Can you work these out from the model? Positions are in its coordinate system, mm. Give positions to 0.01 mm unless a question says otherwise; leave off trailing zeros. Loops run counter-clockwise (first coordinate to the right, second up) from the corner with the lowest first, then second, coordinate; pieces in that order, holes last. Notation, with made-up numbers: M 58,27.5 L 74,27.5 A9 ccw 74,32.5 Z; hole C -1.75,83.25 d7. An arc over 180 degrees is marked long. One line per item, written item: value. Start each with the question number.
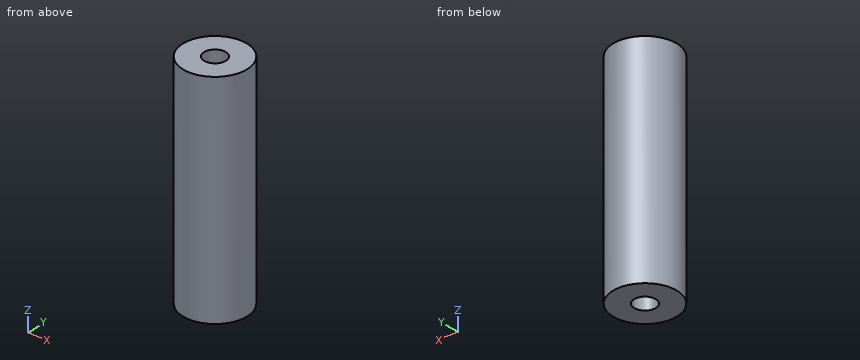
from build123d import *

# Parameters (mm, degrees)
SKETCH_2_W             = 43
SKETCH_2_H             = 12.5
HOLE_WIZARD_M101_D     = 8.5
HOLE_WIZARD_M101_DEPTH = 27.5
HOLE_WIZARD_M101_TIP   = 2.553657631


with BuildPart() as part:
    # Эскиз2 → Повернуть1 (revolve)
    with BuildSketch(Plane(origin=(0, 0, 0), x_dir=(0, 0, -1), z_dir=(1, 0, 0))):
        with Locations((21.5, 6.25)):
            Rectangle(SKETCH_2_W, SKETCH_2_H)
    revolve(axis=Axis((0, 0, 0), (0, 0, -1)))

    # Отверстие обработанное метчиком M101
    with Locations(Plane(origin=(0, 0, -43), x_dir=(-1, 0, 0), z_dir=(0, 0, -1))):
        with Locations((0, 0)):
            Hole(HOLE_WIZARD_M101_D / 2, depth=HOLE_WIZARD_M101_DEPTH)
            with Locations((0, 0, -(HOLE_WIZARD_M101_DEPTH + HOLE_WIZARD_M101_TIP / 2))):  # 118° drill point
                Cone(0, HOLE_WIZARD_M101_D / 2, HOLE_WIZARD_M101_TIP, mode=Mode.SUBTRACT)

    # Зеркальное отражение1: part across plane


with BuildPart() as part_1:
    add(part.part)
    add(part.part.mirror(Plane(origin=(0, 0, 0), x_dir=(1, 0, 0), z_dir=(0, 0, -1))))


solid = part_1.part
Q1. If we section it at B-B, the plane z = 24: Write out the boundary of the cut face in (x, y).
Q2. If we section it at D-D, the plane x = -9: Write out the boundary of the cut face in (y, z), plus the area to 3 significant figures.
Q3. I need wall thicknesses on line 1 along X through (y, z) = (0, 33); line 2 along X through (y, z) = (3.25, -32); line 3 along Y through (x, z) = (-0.5, 3.5). Which ranges of each line are inside material? Lowest first, please.
Q4. If we section it at A-A, the plane z = -1.5: Write out the boundary of the cut face in (x, y), plus the area to 3 significant figures.
Q5. For P1, Ø10, axis at x = 7, z = -8.5, coming from the -Y side; P2, Ø10, axis at y = -7.5, z = 19, coming from the -X side; P3, Ø3, axis at y = 4.5, z = 18.5, coming from the -X side, each with a flat end and sliding along its axis, tell me the tip position at first contact or that it passes through.
Q6. If we section it at C-C, the plane y = 9.5: Write out the boundary of the cut face in (x, z), plus the area to 3 significant figures.
Response:
1. outline: C 0,0 d25; hole C 0,0 d8.5
2. outline: M -8.67,-43 L 8.67,-43 L 8.67,43 L -8.67,43 Z
2. area: 1,490 mm^2
3. line 1: -12.5 to -4.25, 4.25 to 12.5
3. line 2: -12.07 to -2.74, 2.74 to 12.07
3. line 3: -12.49 to 12.49
4. outline: C 0,0 d25
4. area: 491 mm^2
5. P1: y = -12.34
5. P2: x = -12.25
5. P3: x = -12.13
6. outline: M -8.12,-43 L 8.12,-43 L 8.12,43 L -8.12,43 Z
6. area: 1,400 mm^2
